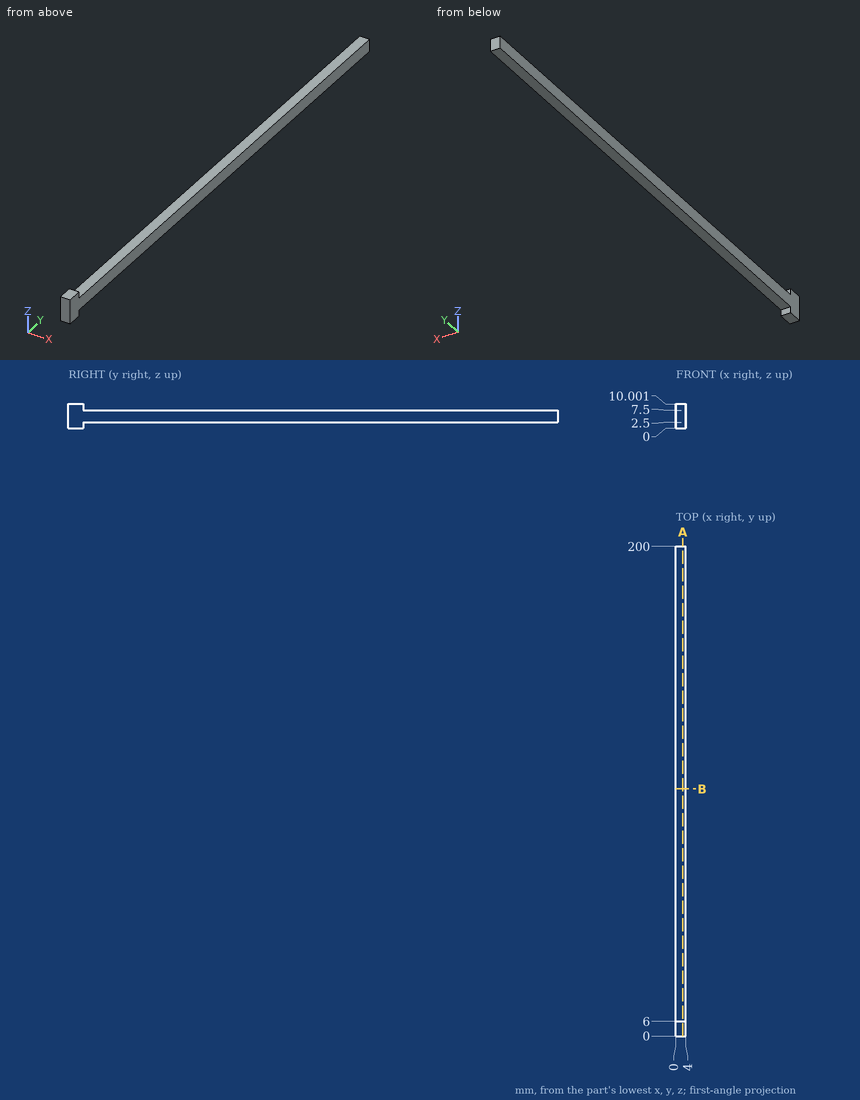
Geometry check sheet. Reference: drawing and pictorial views, mm from the part's lowest x, y, z. Coordinates: 2 decimals unless noted, no trailing zeros. Order: outer loops, then holes, each group sorted by start corner. A loop starts at its lowest first (then second) coordinate and runs counter-clockwise, first axis right, second up.
Item 1: Section check B-B (y = 101). Enter the section's corners in (x, z), plus the area to 3 significant figures.
Item 2: Depth check by flat-ended pin: pin 1 (2 mm diameter, centred on x = 2.5, y = 103, fed in from +Z); pin 2 (1.2 mm diameter, centred on x = 2.5, y = 76, fed in from -Z). Enter the tip coordinate at first touch or a pass-through.
Item 3: Section check A-A (x = 2.9). Enter the section's corners in (y, z), plus the area to 3 significant figures.
Item 4: Scan lines: line 1 along Z through (x, y) = (2.3, 32); line 2 along Y through (x, z) = (1.3, 8.5). Record each from-to range of solid material in increasing order.
Check sheet entries:
1. outline: (0, 2.5) - (4, 2.5) - (4, 7.5) - (0, 7.5) - close
1. area: 20.0 mm2
2. pin 1: stops at z = 7.5
2. pin 2: stops at z = 2.5
3. outline: (0, 0) - (6, 0) - (6, 2.5) - (200, 2.5) - (200, 7.5) - (6, 7.5) - (6, 10) - (0, 10) - close
3. area: 1,030 mm2
4. line 1: z = 2.5 to 7.5
4. line 2: y = 0 to 6
